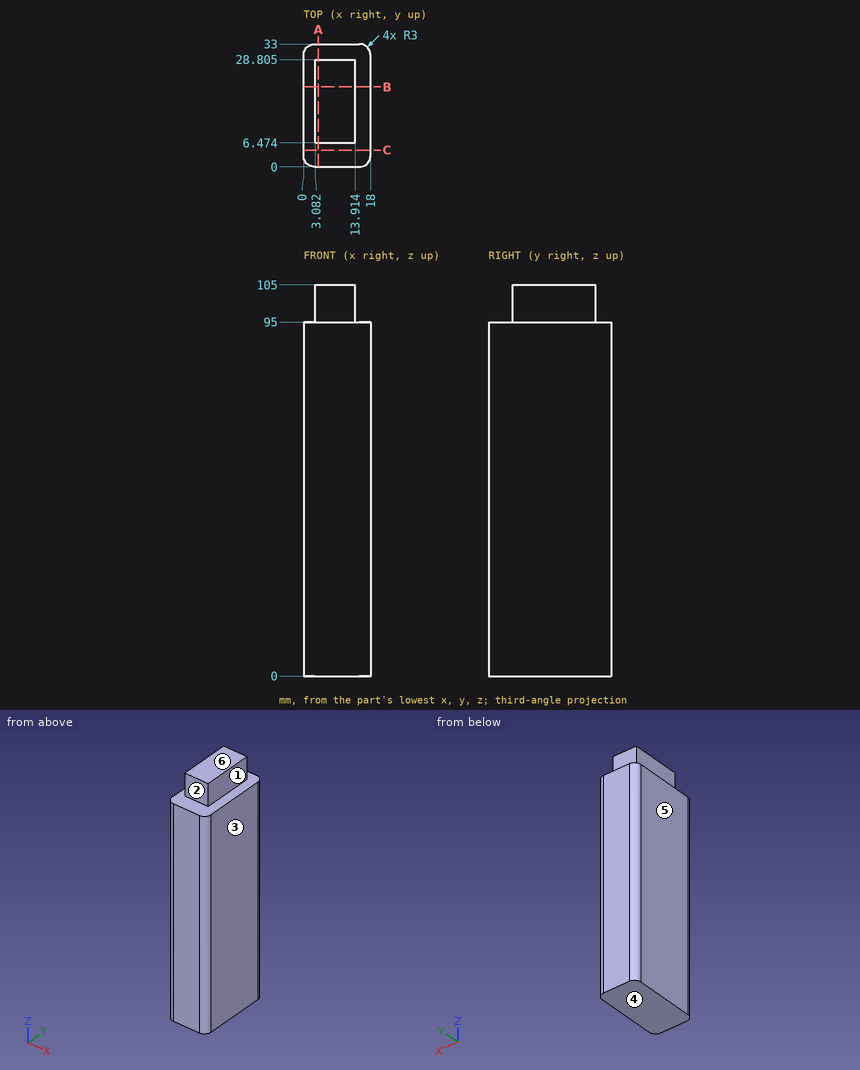
Source: three-view drawing plus pictorial views. Frame: mm from the lowest corner of the part. A direction names the side the tool comes from. Give positions to 0.01 mm unless a question says otherwise; leave off trailing zeros. Order: outer loops, then holes, each group sorted by start corner. A loop starts at its lowest first (then second) coordinate and runs counter-clockwise, first axis right, second up. Notation, with made-up numbers: (69, 50.5) - (121, 50.5) arc R17 ccw to (121, 71.5) - close; hole circle Ø5 at (-9.75, 61). An arc over 180 degrees is marked (long way). Answer as a JSON object with one key per item and string values. Group by question number.
Q1. Set-up query: the marked faces 1, 2 and 3. Return all of +Z, -Z, +X, -X, +Y, -Y with unobstructed straight access to the full face (end or side cutting, diameter ignored); none if empty.
Q2. Line query: probe 1 along Z at (x, y) = (14.5, 23); probe 2 along Y at (x, z) = (16.5, 78); probe 3 along Y at (x, z) = (16.25, 92). Output: solid intervals per line, ascending.
Q3. First-contact query: pin 1 Ø8 at (x, z) = (11, 101.5) entering from -Y; pin 2 Ø8 at (x, z) = (7, 100.5) entering from +Y (1 decimal). Flat tips, straight axial feed; report the tip coordinate or a pass-through.
Q4. Cut plane C-C, the plane y = 4.5. Output: boundary loops of the cut face in (x, z).
Q5. Mould query, pull axis Z, two halves, no side actions, for the marked faces 4, 5 and 6. Classes: pulls with the +Z half, pulls with the -Z half, needs draft (parallel to the pull), parting line crosses it, or undercut.
Q6. Cut plane A-A, the plane x = 4. Output: boundary loops of the cut face in (y, z) (1 decimal), then the cut area to 3 significant figures.
Q7. Cut plane B-B, the plane y = 21.5. Output: boundary loops of the cut face in (x, z) (1 decimal), then the cut area to 3 significant figures.
Results:
{
 "1": {"face 1": "+Z, +X, +Y, -Y", "face 2": "+Z, +X, -X, -Y", "face 3": "+Z, -Z, +X, +Y, -Y"},
 "2": {"probe 1": "0 to 95", "probe 2": "0.4 to 32.6", "probe 3": "0.27 to 32.73"},
 "3": {"pin 1": "y = 6.47", "pin 2": "y = 28.8"},
 "4": {"outline": "(0, 0) - (18, 0) - (18, 95) - (0, 95) - close"},
 "5": {"face 4": "pulls with the -Z half", "face 5": "needs draft", "face 6": "pulls with the +Z half"},
 "6": {"outline": "(0, 0) - (33, 0) - (33, 95) - (28.8, 95) - (28.8, 105) - (6.5, 105) - (6.5, 95) - (0, 95) - close", "area": "3,360 mm^2"},
 "7": {"outline": "(0, 0) - (18, 0) - (18, 95) - (13.9, 95) - (13.9, 105) - (3.1, 105) - (3.1, 95) - (0, 95) - close", "area": "1,820 mm^2"}
}
